Part model, mm, in its own coordinate system. Give positions to 0.01 mm unless a question says otherwise; leave off trailing zeros. Order: outer loops, then holes, each group sorted by start corner. A loop starts at its lowest first (then second) coordinate and runs counter-clockwise, first axis right, second up. Notation, with made-up numbers: (38, -4.75) - (61, -4.75) arc R28 ccw to (61, 29.25) - close; hole circle Ø7 at (38.25, 63.25). An arc over 180 degrees is marked (long way). Use one line per item in the form item = value. Start each with the question number.
1. Band-saw the part on C-C, the plane x = -132. List the corners of the cut face in (y, z).
2. Band-saw the part on D-D, the plane z = 2.95. State how many separate pieces and enclosed holes the cut face has, plus the area to 3 significant figures.
3. Band-saw the part on B-B, the plane x = -17. List the corners of the cut face in (y, z), plus the area to 3 significant figures.
4. Drill centre lines: line 1 (Y direction, x = -81, z = 1.25); line 2 (Y direction, x = -131.5, z = 0.4); line 3 (X direction, y = -158, z = 2.6). Where is each one in solid material? Low to high.
5. Pin check, flat tips, straight feed: P1, Ø2, axis at y = -23, z = 2.5, coming from the -X side; P2, Ø2, axis at y = -38, z = 2, coming from the +X side; P3, Ø1, axis at x = 0.5, z = 2.5, coming from the -Y side. Stop position of each tip, or through.
6. Band-saw the part on A-A, the plane y = -155. List the corners of the cut face in (x, z).
from build123d import *

# Parameters (mm, degrees)
SKETCH1_W           = 200
SKETCH1_H           = 4
BOSS_EXTRUDE1_DEPTH = 4


with BuildPart() as part:
    # Sketch1 → Boss-Extrude1 (new body)
    with BuildSketch(Plane.XY):
        Polygon((-268.2019237, -98.094032778), (-268.2019237, -219.094032778), (-156.2019237, -219.094032778), (-156.2019237, -119.094032778), (-152.2019237, -119.094032778), (-152.2019237, -69.094032778), (-156.2019237, -69.094032778), (-156.2019237, 30.905967222), (-81.2019237, 30.905967222), (-81.2019237, 26.905967222), (18.7980763, 26.905967222), (18.7980763, 30.905967222), (93.7980763, 30.905967222), (93.7980763, -69.094032778), (89.7980763, -69.094032778), (89.7980763, -119.094032778), (93.7980763, -119.094032778), (93.7980763, -219.094032778), (181.7980763, -219.094032778), (181.7980763, -98.094032778), (177.7980763, -98.094032778), (177.7980763, 101.905967222), (181.7980763, 101.905967222), (181.7980763, 222.905967222), (56.7980763, 222.905967222), (56.7980763, 226.905967222), (-143.2019237, 226.905967222), (-143.2019237, 222.905967222), (-268.2019237, 222.905967222), (-268.2019237, 101.905967222), (-264.2019237, 101.905967222), (-264.2019237, -98.094032778), align=None)
        with Locations((-43.2019237, 66.905967222)):
            Rectangle(SKETCH1_W, SKETCH1_H, mode=Mode.SUBTRACT)
        with Locations((-43.2019237, 180.905967222)):
            Rectangle(SKETCH1_W, SKETCH1_H, mode=Mode.SUBTRACT)
    extrude(amount=BOSS_EXTRUDE1_DEPTH)


solid = part.part
From the geometry:
q1.outline = (30.91, 0) - (64.91, 0) - (64.91, 4) - (30.91, 4) - close; (68.91, 0) - (178.91, 0) - (178.91, 4) - (68.91, 4) - close; (182.91, 0) - (226.91, 0) - (226.91, 4) - (182.91, 4) - close
q2.separate_pieces = 1
q2.enclosed_holes = 2
q2.area = 135,000 mm²
q3.outline = (26.91, 0) - (64.91, 0) - (64.91, 4) - (26.91, 4) - close; (68.91, 0) - (178.91, 0) - (178.91, 4) - (68.91, 4) - close; (182.91, 0) - (226.91, 0) - (226.91, 4) - (182.91, 4) - close
q3.area = 768 mm²
q4.line_1 = 26.91 to 64.91, 68.91 to 178.91, 182.91 to 226.91
q4.line_2 = 30.91 to 64.91, 68.91 to 178.91, 182.91 to 226.91
q4.line_3 = -268.2 to -156.2, 93.8 to 181.8
q5.P1 = -264.2
q5.P2 = 177.8
q5.P3 = 26.91
q6.outline = (-268.2, 0) - (-156.2, 0) - (-156.2, 4) - (-268.2, 4) - close; (93.8, 0) - (181.8, 0) - (181.8, 4) - (93.8, 4) - close
